Here's how the part is built. I have some questions about the finished solid (model axes, mm). Give positions to 0.01 mm unless a question says otherwise; leave off trailing zeros. Order: outer loops, then holes, each group sorted by start corner. A loop starts at its lowest first (then second) coordinate and runs counter-clockwise, first axis right, second up. Notation, with made-up numbers: (24.5, -33.5) - (40.5, -33.5) arc R25 cw to (40.5, -21.5) - close; hole circle Ø3 at (33, 49). An arc over 180 degrees is marked (long way). One line per question, with ' | ' between items.
Autodesk Inventor part; units mm, degrees
ref_plane "YZ Plane" through (0, 0, 0) normal (1, 0, 0) x (0, 1, 0)
ref_plane "XZ Plane" through (0, 0, 0) normal (0, 1, 0) x (-1, 0, 0)
ref_plane "XY Plane" through (0, 0, 0) normal (0, 0, 1) x (1, 0, 0)
sketch "Sketch1" plane through (0, 0, 0) normal (0, 0, 1) x (1, 0, 0)
  line L0 (914.4, -2482.85) -> (914.4, 2393.95)
  line L1 (-914.4, 0) -> (914.4, 0)
  line L2 (-914.4, 2393.95) -> (-914.4, -2482.85)
  line L3 (-914.4, 781.05) -> (914.4, 781.05)
  line L4 (-914.4, 732.7159) -> (801.2274, 0)
  line L5 (914.4, 48.3341) -> (-801.2274, 781.05)
  line L6 (914.4, 48.3341) -> (914.4, 0)
  line L7 (801.2274, 0) -> (914.4, 0)
  line L8 (-914.4, 732.7159) -> (-914.4, 781.05)
  line L9 (-801.2274, 781.05) -> (-914.4, 781.05)
  point P0 (0, 0)
extrude "Extrusion1" add sketch "Sketch1" against normal blind 38.1 contours L1 L4 L2 L3 L5 L0
properties part number "side3"
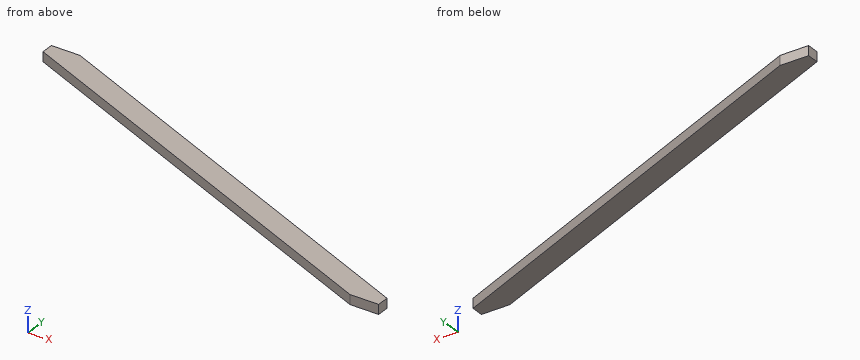
1) I want a section at A-A (z = -31). List the corners of the cut face in (x, y) for me, plus the area to 3 significant figures.
Model answer:
outline: (-914.4, 732.72) - (801.23, 0) - (914.4, 0) - (914.4, 48.33) - (-801.23, 781.05) - (-914.4, 781.05) - close | area: 171,000 mm2
2) I want a section at C-C (y = 415.5). List the corners of the cut face in (x, z) for me.
Model answer:
outline: (-171.65, -38.1) - (54.69, -38.1) - (54.69, 0) - (-171.65, 0) - close
3) I want a section at B-B (x = 308). List the corners of the cut face in (y, z) for me, plus the area to 3 significant figures.
Model answer:
outline: (210.65, -38.1) - (307.32, -38.1) - (307.32, 0) - (210.65, 0) - close | area: 3,680 mm2
4) Please list where these lines run through material, in increasing order: L1, parallel to X at y = 385, z = -11; L2, parallel to X at y = 638, z = -2; L3, parallel to Y at x = 731.5, z = -8.5.
Model answer:
L1: x = -100.24 to 126.11 | L2: x = -692.63 to -466.28 | L3: y = 29.78 to 126.45
5) I'm going to push flat-ended pins straight in: P1, Ø6, axis at x = -213, z = -26.5, coming from the -Y side; P2, Ø1.5, axis at y = 661, z = -14.5, coming from the +X side; P3, Ø1, axis at y = 97, z = -16.5, coming from the +X side. Where does each tip first touch, or does it pass through?
Model answer:
P1: stops at y = 431.88 | P2: stops at x = -518.38 | P3: stops at x = 801.62
